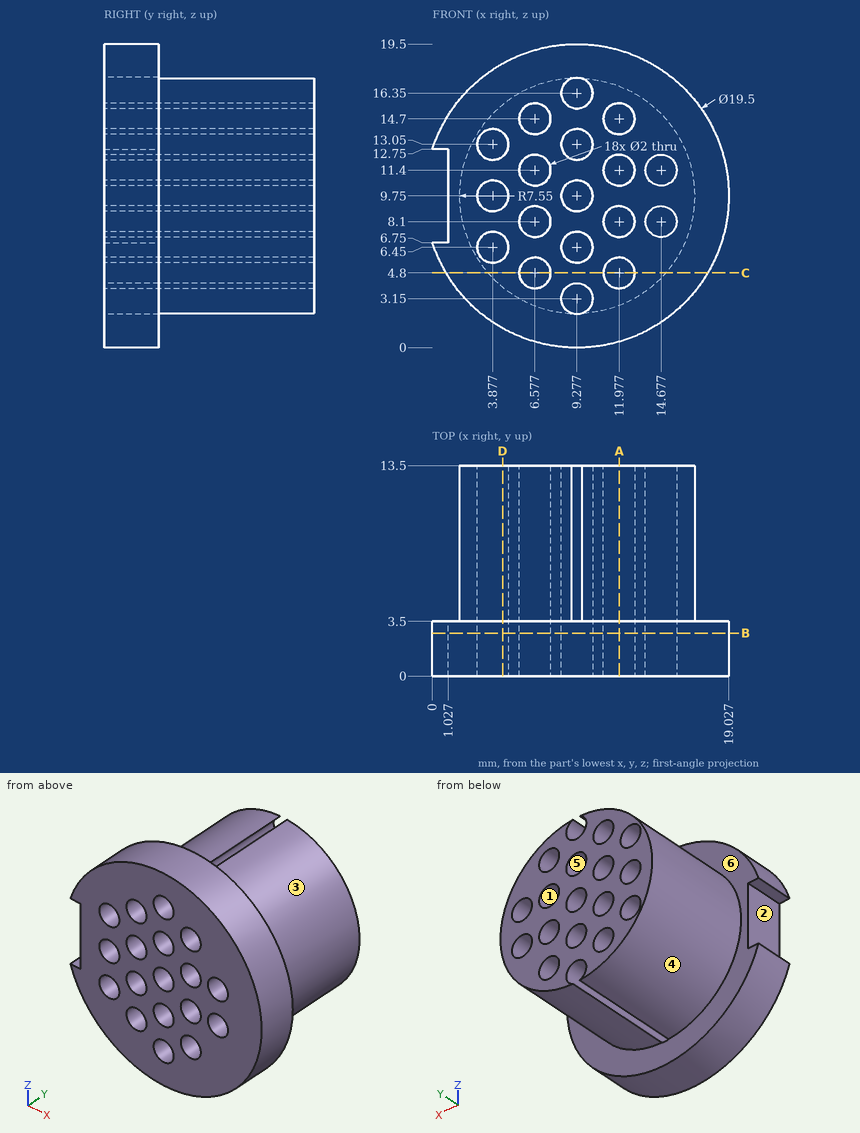
The drawing under review shows one solid part. Ordinate dimensions are in mm from its lowest x, y, z. A direction names the side the tool comes from. Round coordinates to 2 decimals unless told otherwise and drop trailing zeros. Loops run counter-clockwise (first coordinate to the right, second up) from the corner with the lowest first, then second, coordinate; pieces in that order, holes last. Notation, with made-up numbers: (19.5, 80) - (35.5, 80) arc R27 cw to (35.5, 96) - close; hole circle Ø10 at (89.5, 7.5). An arc over 180 degrees is marked (long way). One line per question, with ' | ' between items.
1. We need section A-A, the plane x = 12. State the section outline as (y, z) points, and give its area (3 significant figures).
Results are:
outline: (0, 0.39) - (3.5, 0.39) - (3.5, 2.71) - (13.5, 2.71) - (13.5, 3.8) - (0, 3.8) - close; (0, 5.8) - (13.5, 5.8) - (13.5, 7.1) - (0, 7.1) - close; (0, 9.1) - (13.5, 9.1) - (13.5, 10.4) - (0, 10.4) - close; (0, 12.4) - (13.5, 12.4) - (13.5, 13.7) - (0, 13.7) - close; (0, 15.7) - (13.5, 15.7) - (13.5, 16.79) - (3.5, 16.79) - (3.5, 19.11) - (0, 19.11) - close | area: 98.4 mm²
2. We need section D-D, the plane x = 4.5. State the section outline as (y, z) points.
Results are:
outline: (0, 1.25) - (3.5, 1.25) - (3.5, 3.9) - (13.5, 3.9) - (13.5, 5.67) - (0, 5.67) - close; (0, 7.23) - (13.5, 7.23) - (13.5, 8.97) - (0, 8.97) - close; (0, 10.53) - (13.5, 10.53) - (13.5, 12.27) - (0, 12.27) - close; (0, 13.83) - (13.5, 13.83) - (13.5, 15.6) - (3.5, 15.6) - (3.5, 18.25) - (0, 18.25) - close
3. We need section C-C, the plane z = 4.8. State the section outline as (x, y) points, and give its area (3 significant figures).
Results are:
outline: (0.88, 0) - (5.58, 0) - (5.58, 13.5) - (3.58, 13.5) - (3.58, 3.5) - (0.88, 3.5) - close; (7.58, 0) - (10.98, 0) - (10.98, 13.5) - (7.58, 13.5) - close; (12.98, 0) - (17.68, 0) - (17.68, 3.5) - (14.98, 3.5) - (14.98, 13.5) - (12.98, 13.5) - close | area: 119 mm²
4. We need section B-B, the plane y = 2.75. State how many separate pieces and enclosed holes the cut face has, and give its area (3 significant figures).
Results are:
separate pieces: 1 | enclosed holes: 18 | area: 234 mm²
5. Draft analysis for pull direction Z (two halves, no side actions). For the marked faces 4, 5 and 6, state which applies: released by +Z, released by -Z, zero draft, split by the parting line, or undercut.
Results are:
face 4: split by the parting line | face 5: undercut | face 6: zero draft
6. Clearance check with flat-ended pins moving along their axes: P1, Ø0.5, axis at x = 0.5, y = 2, coming from the -Z side; P2, Ø1.5, axis at y = 6, z = 3, coming from the +X side; P3, Ø3, axis at y = 9, z = 4, coming from the +X side. State where each tip first meets the part, or that it passes through.
Results are:
P1: stops at z = 5.02 | P2: stops at x = 13.86 | P3: stops at x = 15.52
7. For L1, parallel to Z at x = 9.5, y = 1.75; L2, parallel to Z at x = 5.75, y = 10.25; L3, parallel to X at y = 12, z = 15.5, list the stretches that pass through material, from the lowest coordinate up. Write a range as [from, to].
Results are:
L1: z = [0, 2.18], [4.12, 5.48], [7.42, 8.78], [10.72, 12.08], [14.02, 15.38], [17.32, 19.5] | L2: z = [3.07, 4.24], [5.36, 7.54], [8.66, 10.84], [11.96, 14.14], [15.26, 16.43] | L3: x = [4.38, 5.98], [7.18, 8.75], [9.8, 11.38], [12.58, 14.17]
8. For the marked faces 1, 2 and 3, list the 3-axis set-ups (+Z, -Z, +X, -X, +Y, -Y) from which the entire face can be reached by the end or side of a thin tool; tool diameter is ignored.
Results are:
face 1: +Y, -Y | face 2: -X, +Y, -Y | face 3: +X, +Y
